The listing builds one solid part. Answer for the finished solid, in the listing's coordinates (mm). A direction names the side the tool comes from. Round coordinates to 2 decimals unless told otherwise and drop trailing zeros. Order: outer loops, then holes, each group sorted by start corner. A loop starts at its lowest first (then second) coordinate and runs counter-clockwise, first axis right, second up. Notation, with made-up numbers: (-26, 83.5) - (7, 83.5) arc R25 ccw to (7, 108.5) - close; hole circle Ø4 at (24, 3.25). An arc over 180 degrees is marked (long way). Use CSV: the item, a comma, the result in double quotes. Start each with the question number.
Item 1: Find section A-A, the plane x = 31.75. Give the vertices of the cut face in (y, z).
Item 2: Straight lines are drawn through the part: line 1 along X through (y, z) = (6.75, -3); line 2 along Y through (x, z) = (-31.75, 13.5); line 3 along Z through (x, y) = (-29, 0.75). For each, find the intervals that lie inside material, in ascending order. Write a range as [from, to].
Item 3: Find section B-B, the plane y = 6.35. Count the separate pieces of the cut face and the enclosed holes in it, plus the area to 3 significant figures.
Item 4: Flat-ended cylindrical pins translate along their axes: P1, Ø3, axis at y = 2.5, z = -11, coming from the +X side; P2, Ø6, axis at y = 8.5, z = 12.5, coming from the -X side; P3, Ø4, axis at y = 8, z = 0.5, coming from the -X side. Find the tip coordinate at first contact, or state that the pin passes through.
Item 5: Find section D-D, the plane x = -32. Give the vertices of the cut face in (y, z).
Item 6: Determine the mould class of faces 4 (the flat face through (19.05, 6, 0)), 5 (the flat face through (-27, 6, -16.7)), 6 (the cylindrical face through (31.42, 8.83, 14.67)) for opening direction Z: +Z half, -Z half, draft (parallel to the pull), parting line (faces both ways), or undercut.
Item 7: Find section C-C, the plane x = 22. Give the vertices of the cut face in (y, z), plus the area to 3 significant figures.
Item 8: For faces 1 (the cylindrical face through (-9.78, 6.44, 16.49)), 2 (the flat face through (8.744, 6.261, 3.728)), 3 (the cylindrical face through (-9.78, 6.44, -16.49)), determine the directions among +Z, -Z, +X, -X, +Y, -Y from which every point of the face is accessible in a straight line to the end or side of a thin tool.
```python
from build123d import *

# Parameters (mm, degrees)
BOSS_EXTRUDE1_DEPTH     = 12.7
FILLET1_R               = 2.54
SKETCH3_R               = 2.5
CUT_EXTRUDE1_DEPTH      = 30.4
CUT_EXTRUDE1_DEPTH_BACK = 5


with BuildPart() as part:
    # Sketch1 → Boss-Extrude1 (new body)
    with BuildSketch(Plane(origin=(0, 0, 0), x_dir=(1, 0, 0), z_dir=(0, 1, 0))):
        Polygon((-19.05, -12.7), (-19.05, 12.7), (-44.45, 12.7), (-44.45, 16.7), (-9.665344582, 16.7), (0, 5.974999699), (9.665344582, 16.7), (44.45, 16.7), (44.45, 12.7), (19.05, 12.7), (19.05, -12.7), (44.45, -12.7), (44.45, -16.7), (9.665344582, -16.7), (0, -5.974999699), (-9.665344582, -16.7), (-44.45, -16.7), (-44.45, -12.7), align=None)
        Polygon((-15.05, -10.725000301), (-15.05, 10.725000301), (-5.384655418, 0), align=None, mode=Mode.SUBTRACT)
        Polygon((15.05, -10.725000301), (15.05, 10.725000301), (5.384655418, 0), align=None, mode=Mode.SUBTRACT)
    extrude(amount=BOSS_EXTRUDE1_DEPTH)

    # Fillet1
    fillet1_edges = [part.edges().sort_by_distance(p)[0] for p in [
        (-44.45, 6.35, -16.7),
        (-9.665344582, 6.35, -16.7),
        (0, 6.35, -5.974999699),
        (9.665344582, 6.35, -16.7),
        (44.45, 6.35, -16.7),
        (44.45, 6.35, 16.7),
        (9.665344582, 6.35, 16.7),
        (0, 6.35, 5.974999699),
        (-9.665344582, 6.35, 16.7),
        (-44.45, 6.35, 16.7),
        (-15.05, 6.35, 10.725000301),
        (-5.384655418, 6.35, 0),
        (-15.05, 6.35, -10.725000301),
        (5.384655418, 6.35, 0),
        (15.05, 6.35, 10.725000301),
        (15.05, 6.35, -10.725000301),
    ]]
    fillet(fillet1_edges, radius=FILLET1_R)

    # Sketch3 → Cut-Extrude1 (cut, two sides)
    with BuildSketch(Plane.XY.offset(-12.7)) as cut_extrude1_sk:
        with Locations((-31.75, 6.35)):
            Circle(SKETCH3_R)
        with Locations((31.75, 6.35)):
            Circle(SKETCH3_R)
    extrude(amount=CUT_EXTRUDE1_DEPTH, mode=Mode.SUBTRACT)
    extrude(cut_extrude1_sk.sketch, amount=-CUT_EXTRUDE1_DEPTH_BACK, mode=Mode.SUBTRACT)


solid = part.part
```
Worked out:
1,outline,"(0, -16.7) - (3.85, -16.7) - (3.85, -12.7) - (0, -12.7) - close; (0, 12.7) - (3.85, 12.7) - (3.85, 16.7) - (0, 16.7) - close; (8.85, -16.7) - (12.7, -16.7) - (12.7, -12.7) - (8.85, -12.7) - close; (8.85, 12.7) - (12.7, 12.7) - (12.7, 16.7) - (8.85, 16.7) - close"
2,line 1,"x = [-19.05, -15.05], [-8.09, 8.09], [15.05, 19.05]"
2,line 2,"y = [0, 3.85], [8.85, 12.7]"
2,line 3,"z = [-16.7, -12.7], [12.7, 16.7]"
3,separate pieces,"5"
3,enclosed holes,"2"
3,area,"1,220 mm²"
4,P1,"stops at x = 19.05"
4,P2,"stops at x = -44.45"
4,P3,"stops at x = -19.05"
5,outline,"(0, -16.7) - (3.86, -16.7) - (3.86, -12.7) - (0, -12.7) - close; (0, 12.7) - (3.86, 12.7) - (3.86, 16.7) - (0, 16.7) - close; (8.84, -16.7) - (12.7, -16.7) - (12.7, -12.7) - (8.84, -12.7) - close; (8.84, 12.7) - (12.7, 12.7) - (12.7, 16.7) - (8.84, 16.7) - close"
6,face 4,"undercut"
6,face 5,"-Z half"
6,face 6,"draft"
7,outline,"(0, -16.7) - (12.7, -16.7) - (12.7, -12.7) - (0, -12.7) - close; (0, 12.7) - (12.7, 12.7) - (12.7, 16.7) - (0, 16.7) - close"
7,area,"102 mm²"
8,face 1,"+Z, +Y, -Y"
8,face 2,"+Y, -Y"
8,face 3,"-Z, +Y, -Y"
